Design review of the part built by this model. Coordinates are the model's own, in mm. Coordinates: 2 decimals unless noted, no trailing zeros. Loops run counter-clockwise (first coordinate to the right, second up) from the corner with the lowest first, then second, coordinate; pieces in that order, holes last.
Q1. Add section C-C on x = 100. Give the boundary of the cut face in (y, z).
Q2. Wall thickness on probe 1 along Y at (x, z) = (100, 4.4); probe 2 along X at (y, z) = (102, 3.4); probe 3 along Y at (x, z) = (20, 4.15): over which ranges is each line inside the solid? List them lowest first.
Q3. Add section B-B on y = 100. Give the boundary of the cut face in (x, z).
Q4. Add section A-A on x = 20. Give the boundary of the cut face in (y, z), and give its area (3 significant figures).
Q5. Draft analysis for pull direction Y (two halves, no side actions). For faces 1 (the face through (99, 200, 3)), 2 (the face through (20.65, 97.07, 2.96)), 3 (the face through (76, 101, 0)), state which applies: released by +Y, released by -Y, zero draft, split by the parting line, or undercut.
```python
from build123d import *

# Parameters (mm, degrees)
F0_W     = 200
F0_H     = 200
F1_DEPTH = 6
F3_D     = 6
F5_D     = 25


with BuildPart() as f1:
    # F0 (on Top) → F1 (new body)
    with BuildSketch(Plane.XY):
        with Locations((100, 100)):
            Rectangle(F0_W, F0_H)
    extrude(amount=F1_DEPTH)

    # F3 (through all)
    with Locations(Plane.XY.offset(6)):
        with Locations((20, 100), (180, 100)):
            Hole(F3_D / 2)

    # F5 (through all)
    with Locations(Plane.XY.offset(6)):
        with Locations((100, 100)):
            Hole(F5_D / 2)


solid = f1.part
```
Entries:
1. outline: (0, 0) - (87.5, 0) - (87.5, 6) - (0, 6) - close; (112.5, 0) - (200, 0) - (200, 6) - (112.5, 6) - close
2. probe 1: y = 0 to 87.5, 112.5 to 200
2. probe 2: x = 0 to 17.76, 22.24 to 87.66, 112.34 to 177.76, 182.24 to 200
2. probe 3: y = 0 to 97, 103 to 200
3. outline: (0, 0) - (17, 0) - (17, 6) - (0, 6) - close; (23, 0) - (87.5, 0) - (87.5, 6) - (23, 6) - close; (112.5, 0) - (177, 0) - (177, 6) - (112.5, 6) - close; (183, 0) - (200, 0) - (200, 6) - (183, 6) - close
4. outline: (0, 0) - (97, 0) - (97, 6) - (0, 6) - close; (103, 0) - (200, 0) - (200, 6) - (103, 6) - close
4. area: 1,160 mm2
5. face 1: released by +Y
5. face 2: undercut
5. face 3: zero draft
